Read the model definition and answer for the solid it produces. Units are mm, in the model's axes. Face numbers are marked on the shaded views. A direction names the side the tool comes from. Coordinates: 2 decimals unless noted, no trailing zeros. Loops run counter-clockwise (first coordinate to the right, second up) from the corner with the lowest first, then second, coordinate; pieces in that order, holes last. Notation, with made-up numbers: (-40, -4) -> (-25, -4) arc R9 ccw to (-25, 6) -> close; hole circle Ø5 at (15.25, 77.25). An arc over 180 degrees is marked (long way). Answer in a Markdown table with one row per item.
```python
from build123d import *

# Parameters (mm, degrees)
F0_W     = 23.5
F0_H     = 3
F1_DEPTH = 3
F2_DEPTH = 20
F3_R     = 2.5


with BuildPart() as f1:
    # F0 (on Top) → F1 (new body)
    with BuildSketch(Plane.XY):
        Polygon((-14.5, 24.875), (-14.5, -15.625), (-7.5, -15.625), (-7.5, -10.125), (-4.5, -10.125), (19, -10.125), (19, -6.125), (19, 24.875), align=None)
        Polygon((-7.5, -15.625), (-14.5, -15.625), (-14.5, -18.625), (-7.5, -18.625), (-4.5, -18.625), (-4.5, -13.125), (-4.5, -10.125), (-7.5, -10.125), align=None)
        with Locations((7.25, -11.625)):
            Rectangle(F0_W, F0_H)
        Polygon((22, -6.125), (19, -6.125), (19, -10.125), (19, -13.125), (22, -13.125), (22, -10.125), align=None)
    extrude(amount=-F1_DEPTH)

    # F0 (on Top) → F2 (join)
    with BuildSketch(Plane.XY):
        Polygon((22, -6.125), (19, -6.125), (19, -10.125), (19, -13.125), (22, -13.125), (22, -10.125), align=None)
        with Locations((7.25, -11.625)):
            Rectangle(F0_W, F0_H)
        Polygon((-7.5, -15.625), (-14.5, -15.625), (-14.5, -18.625), (-7.5, -18.625), (-4.5, -18.625), (-4.5, -13.125), (-4.5, -10.125), (-7.5, -10.125), align=None)
    extrude(amount=F2_DEPTH)

    # F3
    f3_edges = [f1.edges().sort_by_distance(p)[0] for p in [
        (-14.5, 3.125, -3),
        (-14.5, -18.625, 8.5),
        (-9.5, -18.625, -3),
        (-4.5, -15.875, -3),
        (8.75, -13.125, -3),
        (-4.5, -13.125, 8.5),
        (-4.5, -18.625, 8.5),
        (22, -13.125, 8.5),
        (22, -9.625, -3),
        (8.75, -13.125, 20),
        (-4.5, -15.875, 20),
        (-9.5, -18.625, 20),
        (22, -9.625, 20),
        (22, -6.125, 8.5),
        (20.5, -6.125, -3),
        (19, 9.375, -3),
        (20.5, -6.125, 20),
        (-14.5, -17.125, 20),
    ]]
    fillet(f3_edges, radius=F3_R)


solid = f1.part
```
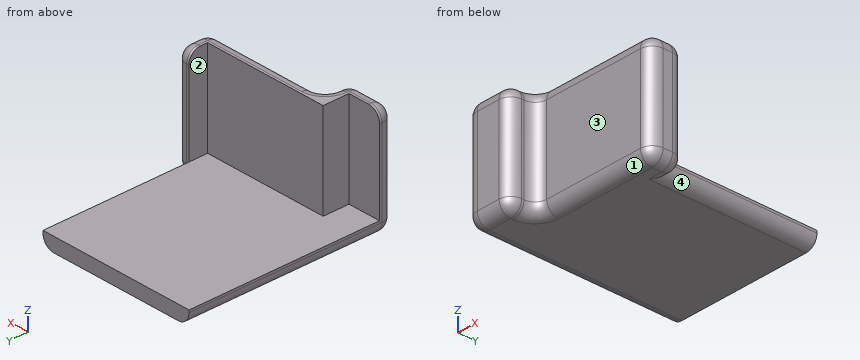
1. A cutting plane is placed at B-B on x = -10. Give the vertices of the cut face in (y, z) (3 decimals).
A:
| item | result |
|---|---|
| outline | (-18.625, -0.5) arc R2.5 ccw to (-16.125, -3) -> (24.875, -3) -> (24.875, 0) -> (-15.625, 0) -> (-15.625, 20) -> (-16.125, 20) arc R2.5 ccw to (-18.625, 17.5) -> close |
2. A cutting plane is placed at D-D on x = 13.5. Give the vertices of the cut face in (y, z) (3 decimals), and give its area (3 significant figures).
A:
| item | result |
|---|---|
| outline | (-13.125, -0.5) arc R2.5 ccw to (-10.625, -3) -> (24.875, -3) -> (24.875, 0) -> (-10.125, 0) -> (-10.125, 20) -> (-10.625, 20) arc R2.5 ccw to (-13.125, 17.5) -> close |
| area | 171 mm2 |
3. A cutting plane is placed at C-C on z = 12.75. Give the vertices of the cut face in (x, y) (3 decimals), and give its area (3 significant figures).
A:
| item | result |
|---|---|
| outline | (-14.5, -16.125) arc R2.5 ccw to (-12, -18.625) -> (-7, -18.625) arc R2.5 ccw to (-4.5, -16.125) -> (-4.5, -15.625) arc R2.5 cw to (-2, -13.125) -> (19.5, -13.125) arc R2.5 ccw to (22, -10.625) -> (22, -8.625) arc R2.5 ccw to (19.5, -6.125) -> (19, -6.125) -> (19, -10.125) -> (-7.5, -10.125) -> (-7.5, -15.625) -> (-14.5, -15.625) -> close |
| area | 134 mm2 |
4. Given pin 1 Ø6 at (x, z) = (4.5, 7) entering from +Y (3 decimals); pin 2 Ø4 at (y, z) = (-3, 9) entering from +X; pin 3 Ø4.5 at (y, z) = (-12, 9) entering from -X; pin 4 Ø1.2 at (y, z) = (-9, 7.5) entering from -X, each flat-ended and moving along its own axis, determine where each tip first touches the part or whether it passes through.
A:
| item | result |
|---|---|
| pin 1 | stops at y = -10.125 |
| pin 2 | passes through |
| pin 3 | stops at x = -7.5 |
| pin 4 | stops at x = 19 |
5. Find the intervals of material crossed by probe 1 along Z at (x, y) = (-1, 20.5); probe 2 along Y at (x, z) = (3, 16.25) (3 decimals); probe 3 along Y at (x, z) = (-9, 13.5) (3 decimals), in increasing order.
A:
| item | result |
|---|---|
| probe 1 | z = -3 to 0 |
| probe 2 | y = -13.125 to -10.125 |
| probe 3 | y = -18.625 to -15.625 |
6. A tool of negligible diameter and unlimited length cuts with its end or side. For the marked faces 1, 2, 3 and 4, from which of +Z, -Z, +X, -X, +Y, -Y can it reach the whole face along a straight path? Write none if from no direction.
A:
| item | result |
|---|---|
| face 1 | -Z, +X, -Y |
| face 2 | +Z, -X, +Y |
| face 3 | +Z, -Z, +X, -Y |
| face 4 | -Z, +X, +Y |
7. A cutting plane is placed at A-A on y = 21. Give the vertices of the cut face in (x, z), and give its area (3 significant figures).
A:
| item | result |
|---|---|
| outline | (-14.5, -0.5) arc R2.5 ccw to (-12, -3) -> (16.5, -3) arc R2.5 ccw to (19, -0.5) -> (19, 0) -> (-14.5, 0) -> close |
| area | 97.8 mm2 |
